Verification items for the finished model (mm, model axes). Give positions to 0.01 mm unless a question says otherwise; leave off trailing zeros. Write each loop counter-clockwise with the first axis right and the second up, starting at its lowest first coordinate (ties: lowest second). Pieces come first, ordered by that corner, then holes. Notation, with made-up numbers: M 26.5,-19.5 L 68.5,-19.5 A22 cw 68.5,8.5 Z; hole C -8.5,84 d1. An arc over 180 degrees is marked long. Write item = value, one per line.
from build123d import *

# Parameters (mm, degrees)
SKETCH1_R           = 3.05
SKETCH1_R_2         = 20.5
BOSS_EXTRUDE1_DEPTH = 2


with BuildPart() as part:
    # Sketch1 → Boss-Extrude1 (new body)
    with BuildSketch(Plane.XY):
        with BuildLine():
            Line((-30, 30), (30, 30))
            ThreePointArc((30, 30), (32.828427125, 28.828427125), (34, 26))
            Line((34, 26), (34, -26))
            ThreePointArc((34, -26), (32.828427125, -28.828427125), (30, -30))
            Line((30, -30), (-30, -30))
            ThreePointArc((-30, -30), (-32.828427125, -28.828427125), (-34, -26))
            Line((-34, -26), (-34, 26))
            ThreePointArc((-34, 26), (-32.828427125, 28.828427125), (-30, 30))
        make_face()
        with Locations((22.5, -22.5)):
            Circle(SKETCH1_R, mode=Mode.SUBTRACT)
        with Locations(Location((-22.5, -22.5, 0), (0, 0, 180))):
            Circle(SKETCH1_R, mode=Mode.SUBTRACT)
        with Locations((-22.5, 22.5)):
            Circle(SKETCH1_R, mode=Mode.SUBTRACT)
        with Locations(Location((22.5, 22.5, 0), (0, 0, 180))):
            Circle(SKETCH1_R, mode=Mode.SUBTRACT)
        Circle(SKETCH1_R_2, mode=Mode.SUBTRACT)
    extrude(amount=BOSS_EXTRUDE1_DEPTH)


solid = part.part
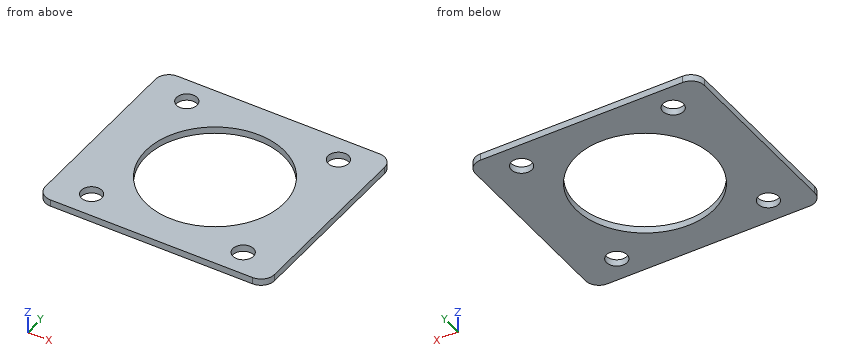
1) Material ranges on probe 1 along Y at (x, z) = (22.5, 1.15); probe 2 along Y at (x, z) = (0.5, 1.45); probe 3 along Y at (x, z) = (-5, 1.3), recorded low to high. Write a range as from..to.
From the geometry:
probe_1 = -30..-25.55, -19.45..19.45, 25.55..30
probe_2 = -30..-20.49, 20.49..30
probe_3 = -30..-19.88, 19.88..30
2) Cross-section at C-C on y = -22.5. Record the boundary of the cut face in (x, z).
From the geometry:
outline = M -34,0 L -25.55,0 L -25.55,2 L -34,2 Z; M -19.45,0 L 19.45,0 L 19.45,2 L -19.45,2 Z; M 25.55,0 L 34,0 L 34,2 L 25.55,2 Z
3) Cross-section at B-B on x = -22.5. Record the boundary of the cut face in (y, z).
From the geometry:
outline = M -30,0 L -25.55,0 L -25.55,2 L -30,2 Z; M -19.45,0 L 19.45,0 L 19.45,2 L -19.45,2 Z; M 25.55,0 L 30,0 L 30,2 L 25.55,2 Z
4) Cross-section at D-D on z = 0.8. Record the boundary of the cut face in (x, y).
From the geometry:
outline = M -34,-26 A4 ccw -30,-30 L 30,-30 A4 ccw 34,-26 L 34,26 A4 ccw 30,30 L -30,30 A4 ccw -34,26 Z; hole C -22.5,-22.5 d6.1; hole C -22.5,22.5 d6.1; hole C 0,0 d41; hole C 22.5,-22.5 d6.1; hole C 22.5,22.5 d6.1
5) Cross-section at A-A on y = 0. Record the boundary of the cut face in (x, z), plus the area to 3 significant figures.
From the geometry:
outline = M -34,0 L -20.5,0 L -20.5,2 L -34,2 Z; M 20.5,0 L 34,0 L 34,2 L 20.5,2 Z
area = 54.0 mm^2
